from build123d import *

# Parameters (mm, degrees)
F0_W     = 101
F0_H     = 91
F1_DEPTH = 5
F3_D     = 12.5
F5_D     = 7


with BuildPart() as f1:
    # F0 (on Top) → F1 (new body)
    with BuildSketch(Plane.XY):
        with Locations((0, -45.5)):
            Rectangle(F0_W, F0_H)
    extrude(amount=-F1_DEPTH)

    # F3 (through all)
    with Locations(Plane.XY):
        with Locations((-40.5, -76), (40.5, -76), (40.5, -15), (-40.5, -15), (0, -45.5)):
            Hole(F3_D / 2)

    # F5 (through all)
    with Locations(Plane(origin=(0, 0, -5), x_dir=(1, 0, 0), z_dir=(0, 0, -1))):
        with Locations((-18.73833, 64.23833), (-18.73833, 26.76167), (18.73833, 26.76167), (18.73833, 64.23833)):
            Hole(F5_D / 2)


solid = f1.part
Verification items for the finished model (mm, model axes). Coordinates: 2 decimals unless noted, no trailing zeros. Write each loop counter-clockwise with the first axis right and the second up, starting at its lowest first coordinate (ties: lowest second). Pieces come first, ordered by that corner, then holes. Notation, with made-up numbers: M 19,-28.75 L 47,-28.75 A13 cw 47,-18.75 Z; hole C -29,-8 d4. An arc over 180 degrees is marked long. Use a Markdown table: item, result.
Q1. Sectioned sample at A-A, the plane x = -40.5. Record the boundary of the cut face in (y, z).
Reply:
| item | result |
|---|---|
| outline | M -91,-5 L -82.25,-5 L -82.25,0 L -91,0 Z; M -69.75,-5 L -21.25,-5 L -21.25,0 L -69.75,0 Z; M -8.75,-5 L 0,-5 L 0,0 L -8.75,0 Z |
Q2. Sectioned sample at D-D, the plane y = -76. Record the boundary of the cut face in (x, z).
Reply:
| item | result |
|---|---|
| outline | M -50.5,-5 L -46.75,-5 L -46.75,0 L -50.5,0 Z; M -34.25,-5 L 34.25,-5 L 34.25,0 L -34.25,0 Z; M 46.75,-5 L 50.5,-5 L 50.5,0 L 46.75,0 Z |
Q3. Sectioned sample at C-C, the plane z = -3.55. Count the separate pieces of the cut face and the enclosed holes in it, plus the area to 3 significant figures.
Reply:
| item | result |
|---|---|
| separate pieces | 1 |
| enclosed holes | 9 |
| area | 8,420 mm² |
Q4. Thickness scan on line 1 (Y direction, x = 40, z = -1.45); line 2 (X direction, y = -12.5, z = -3.8); line 3 (X direction, y = -25.5, z = -3.95). Record the ranges inside material, lowest first.
Reply:
| item | result |
|---|---|
| line 1 | y = -91 to -82.23, -69.77 to -21.23, -8.77 to 0 |
| line 2 | x = -50.5 to -46.23, -34.77 to 34.77, 46.23 to 50.5 |
| line 3 | x = -50.5 to -22, -15.47 to 15.47, 22 to 50.5 |
Q5. Sectioned sample at B-B, the plane y = -45.5. Record the boundary of the cut face in (x, z).
Reply:
| item | result |
|---|---|
| outline | M -50.5,-5 L -6.25,-5 L -6.25,0 L -50.5,0 Z; M 6.25,-5 L 50.5,-5 L 50.5,0 L 6.25,0 Z |
Q6. Draft check along Y on faces 1 (the face through (41.3, -69.8, -2.5)), 2 (the face through (0.8, -39.3, -2.5)), 3 (the face through (-1, 0, -2)), 4 (the face through (-50.5, -46, -2)). Enter one of: +Y half, -Y half, draft (parallel to the pull), parting line (faces both ways), or undercut.
Reply:
| item | result |
|---|---|
| face 1 | undercut |
| face 2 | undercut |
| face 3 | +Y half |
| face 4 | draft |
